```python
from build123d import *

# Parameters (mm, degrees)
BOSS_EXTRUDE2_DEPTH = 10
SKETCH7_R           = 2.5
CUT_EXTRUDE1_DEPTH  = 142.937027035


with BuildPart() as part:
    # Sketch3 → Boss-Extrude2 (new body)
    with BuildSketch(Plane(origin=(0, 0, 0), x_dir=(1, 0, 0), z_dir=(0, 1, 0))):
        with BuildLine():
            ThreePointArc((-5, -49.835383767), (-3.535533906, -46.299849861), (0, -44.835383767))
            ThreePointArc((0, -44.835383767), (3.535533906, -46.299849861), (5, -49.835383767))
            Line((5, -49.835383767), (5, -59.835383767))
            Line((5, -59.835383767), (10, -59.835383767))
            Line((10, -59.835383767), (10, -49.835383767))
            ThreePointArc((10, -49.835383767), (9.713312199, -47.45808149), (8.869686776, -45.217087925))
            ThreePointArc((8.869686776, -45.217087925), (7.18243593, -40.735100795), (6.609060329, -35.98049624))
            Line((6.609060329, -35.98049624), (6.609060329, 120.164616233))
            Line((6.609060329, 120.164616233), (5, 120.164616233))
            Line((5, 120.164616233), (5, 140.164616233))
            Line((5, 140.164616233), (-5, 140.164616233))
            Line((-5, 140.164616233), (-5, 120.164616233))
            Line((-5, 120.164616233), (-7.105716065, 120.164616233))
            Line((-7.105716065, 120.164616233), (-7.105716065, -36.979250733))
            ThreePointArc((-7.105716065, -36.979250733), (-7.594058684, -41.37188391), (-9.035238688, -45.550006089))
            ThreePointArc((-9.035238688, -45.550006089), (-9.755828695, -47.6390672), (-10, -49.835383811))
            Line((-10, -49.835383811), (-10, -59.835383767))
            Line((-10, -59.835383767), (-5, -59.835383767))
            Line((-5, -59.835383767), (-5, -49.835383767))
        make_face()
    extrude(amount=BOSS_EXTRUDE2_DEPTH)

    # Sketch7 → Cut-Extrude1 (cut, through all)
    with BuildSketch(Plane.ZY.offset(10)):
        with BuildLine():
            ThreePointArc((-140.164616233, 5), (-138.700150139, 8.535533906), (-135.164616233, 10))
            Line((-135.164616233, 10), (-140.164616233, 10))
            Line((-140.164616233, 10), (-140.164616233, 5))
        make_face()
        with BuildLine():
            ThreePointArc((-135.164616202, 0), (-138.700150128, 1.464466083), (-140.164616233, 5))
            Line((-140.164616233, 5), (-140.164616233, 0))
            Line((-140.164616233, 0), (-135.164616202, 0))
        make_face()
        with BuildLine():
            ThreePointArc((-135.164616233, 10), (-132.664616233, 9.330127019), (-130.834489214, 7.5))
            Line((-130.834489214, 7.5), (-120.164616233, 7.5))
            Line((-120.164616233, 7.5), (-120.164616233, 10))
            Line((-120.164616233, 10), (-135.164616233, 10))
        make_face()
        with BuildLine():
            Line((-120.164616233, 0), (-120.164616233, 2.5))
            Line((-120.164616233, 2.5), (-130.834489214, 2.5))
            ThreePointArc((-130.834489214, 2.5), (-132.664616219, 0.669872989), (-135.164616202, 0))
            Line((-135.164616202, 0), (-120.164616233, 0))
        make_face()
        Polygon((49.835383767, 2.5), (-120.164616233, 2.5), (-120.164616233, 0), (36.979250733, 0), (45.550006089, 0), (49.835383767, 0), align=None)
        Polygon((-120.164616233, 10), (-120.164616233, 7.5), (49.835383767, 7.5), (49.835383767, 10), (45.550006089, 10), (36.979250733, 10), align=None)
        with BuildLine():
            Line((49.835383767, 10), (49.835383767, 7.5))
            Line((49.835383767, 7.5), (50.675374481, 7.5))
            ThreePointArc((50.675374481, 7.5), (52.5055015, 9.330127019), (55.0055015, 10))
            Line((55.0055015, 10), (49.835383767, 10))
        make_face()
        with BuildLine():
            Line((59.835383767, 10), (55.0055015, 10))
            ThreePointArc((55.0055015, 10), (58.049696739, 8.966468877), (59.835383767, 6.293150141))
            Line((59.835383767, 6.293150141), (59.835383767, 10))
        make_face()
        with BuildLine():
            ThreePointArc((59.835383767, 3.706849859), (58.049696739, 1.033531123), (55.0055015, 0))
            Line((55.0055015, 0), (59.835383767, 0))
            Line((59.835383767, 0), (59.835383767, 3.706849859))
        make_face()
        with BuildLine():
            Line((50.675374481, 2.5), (49.835383767, 2.5))
            Line((49.835383767, 2.5), (49.835383767, 0))
            Line((49.835383767, 0), (55.0055015, 0))
            ThreePointArc((55.0055015, 0), (52.5055015, 0.669872981), (50.675374481, 2.5))
        make_face()
        with Locations((55.0055015, 5)):
            Circle(SKETCH7_R)
        with Locations((-135.164616233, 5)):
            Circle(SKETCH7_R)
    extrude(amount=-CUT_EXTRUDE1_DEPTH, mode=Mode.SUBTRACT)


solid = part.part
```
The model under review builds one solid part; all positions refer to its coordinate system, in mm. A direction names the side the tool comes from. Round coordinates to 2 decimals unless told otherwise and drop trailing zeros. Loops run counter-clockwise (first coordinate to the right, second up) from the corner with the lowest first, then second, coordinate; pieces in that order, holes last. Notation, with made-up numbers: (-6, 71.5) -> (26, 71.5) arc R33 cw to (26, 104.5) -> close; hole circle Ø7 at (62.25, -17.5). An arc over 180 degrees is marked (long way). Answer as a JSON object with one key per item and string values. Group by question number.
1) For pin 1 Ø10 at (x, z) = (4, -89) entering from +Y; pin 2 Ø5 at (y, z) = (2.5, -133.5) entering from -X; pin 3 Ø0.5 at (x, y) = (6, 5.5) entering from -Z, all flat-tipped, find the tip position at first contact; note any pin that passes through.
2) We need section B-B on z = -28. Write out the cut boundary in (x, y), then the cut area to 3 significant figures.
3) We need section A-A on x = 2. Write out the cut boundary in (y, z).
4) For faces 4 (the face through (-5, 5, -130)), 5 (the face through (5, 3.8, 52.5)), 6 (the face through (0, 7.5, -41)), 7 (the face through (6.609, 5, -41)), 8 (the face through (-0.07, 5.11, -137.662)), list the 3-axis set-ups (+Z, -Z, +X, -X, +Y, -Y) from which the entire face can be reached by the end or side of a thin tool; tool diameter is ignored.
5) For line 1 (X direction, y = 4.25, z = 10); line 2 (Y direction, x = -2.5, z = -88); line 3 (Z direction, x = -3, y = 6.75), list the stretches that pass through material, from the lowest coordinate up. Write a range as [from, to].
6) Mouldability with a two-part tool opening along Y and no side actions: class faces 1 (the face through (7.465, 5.11, 52.508)), 2 (the face through (-10, 3.8, 52.5)), 3 (the face through (0, 2.5, -39)) as released by +Y, released by -Y, zero draft, split by the parting line, or undercut.
Result set:
{
 "1": {"pin 1": "y = 7.5", "pin 2": "x = -5", "pin 3": "z = -120.16"},
 "2": {"outline": "(-7.11, 2.5) -> (6.61, 2.5) -> (6.61, 7.5) -> (-7.11, 7.5) -> close", "area": "68.6 mm²"},
 "3": {"outline": "(2.5, -130.83) arc R5 ccw (long way) to (7.5, -130.83) -> (7.5, 45.25) -> (2.5, 45.25) -> close; hole circle Ø5 at (5, -135.16)"},
 "4": {"face 4": "-Z, -X, +Y, -Y", "face 5": "+Z, +Y, -Y", "face 6": "+X, -X, +Y", "face 7": "-Z, +X, +Y, -Y", "face 8": "+X, -X"},
 "5": {"line 1": "[-7.11, 6.61]", "line 2": "[2.5, 7.5]", "line 3": "[-139.85, -136.95], [-133.38, 45.84]"},
 "6": {"face 1": "undercut", "face 2": "zero draft", "face 3": "released by -Y"}
}
